Design review of the part built by this model. Coordinates are the model's own, in mm. A direction names the side the tool comes from. Round coordinates to 2 decimals unless told otherwise and drop trailing zeros. Write each loop counter-clockwise with the first axis right and the second up, starting at its lowest first coordinate (ties: lowest second). Pieces come first, ordered by that corner, then holes. Notation, with made-up numbers: (40, -3.75) -> (45, -3.75) arc R24 cw to (45, 11.25) -> close; hole circle Ø4 at (44, 62). An arc over 180 degrees is marked (long way). One line per question, with ' | ' between items. Start each with the question number.
1) Insertion check: pin 1 Ø1.2 at (y, z) = (5, -8.5) entering from +X; pin 2 Ø3.5 at (x, y) = (-3, 4.5) entering from +Z; pin 3 Ø3.5 at (y, z) = (8, -3) entering from -X. Each pin has a flat end and moves straight along its axis. Give the tip position at first contact, or say it passes through.
2) Consider section C-C (x = 25.4). Give the boundary of the cut face in (y, z).
3) Consider section A-A (y = 6.35). Give the boundary of the cut face in (x, z).
4) Mouldability with a two-part tool opening along Y and no side actions: class faces 5 (the flat face through (-20, 6, -11.049)), 6 (the flat face through (0, 0, -7)), 7 (the cylindrical face through (22.025, 6.499, -12.614)) as +Y half, -Y half, draft (parallel to the pull), parting line (faces both ways), or undercut.
5) Consider section D-D (z = -4.75). Give the boundary of the cut face in (x, y), then the cut area to 3 significant figures.
6) For probe 1 along Y at (x, z) = (25.4, -13.1); probe 2 along X at (y, z) = (7.75, 0); probe 3 along Z at (x, y) = (-1.5, 11.5), list the stretches that pass through material, from the lowest coordinate up.
7) Consider section B-B (x = 0). Give the boundary of the cut face in (y, z), then the cut area to 3 significant figures.
8) For faces 1 (the flat face through (9.271, 6, -6)), 2 (the cylindrical face through (0.2, 6.26, 9.27)), 3 (the flat face through (-9.271, 6, -5)), 4 (the flat face through (-6.096, 6, -9)), list the 3-axis set-ups (+Z, -Z, +X, -X, +Y, -Y) from which the entire face can be reached by the end or side of a thin tool; tool diameter is ignored.
```python
from build123d import *

# Parameters (mm, degrees)
SKETCH1_R           = 6.096
BOSS_EXTRUDE1_DEPTH = 12.7
SKETCH2_R           = 3.3782
CUT_EXTRUDE1_DEPTH  = 4.175


with BuildPart() as part:
    # Sketch1 → Boss-Extrude1 (new body)
    with BuildSketch(Plane(origin=(0, 0, 0), x_dir=(1, 0, 0), z_dir=(0, 1, 0))):
        with BuildLine():
            Line((-9.271, 0), (-9.271, 11.049))
            Line((-9.271, 11.049), (-31.496, 11.049))
            Line((-31.496, 11.049), (-31.496, 14.224))
            Line((-31.496, 14.224), (-6.096, 14.224))
            Line((-6.096, 14.224), (6.096, 14.224))
            Line((6.096, 14.224), (31.496, 14.224))
            Line((31.496, 14.224), (31.496, 11.049))
            Line((31.496, 11.049), (9.271, 11.049))
            Line((9.271, 11.049), (9.271, 0))
            ThreePointArc((9.271, 0), (0, -9.271), (-9.271, 0))
        make_face()
        Circle(SKETCH1_R, mode=Mode.SUBTRACT)
        with BuildLine():
            Line((-6.096, 7.112), (-6.096, 11.049))
            Line((-6.096, 11.049), (6.096, 11.049))
            Line((6.096, 11.049), (6.096, 7.112))
            ThreePointArc((6.096, 7.112), (0, 9.367057169), (-6.096, 7.112))
        make_face(mode=Mode.SUBTRACT)
    extrude(amount=BOSS_EXTRUDE1_DEPTH)

    # Sketch2 → Cut-Extrude1 (cut, through all)
    with BuildSketch(Plane.XY.offset(-11.049)):
        with Locations((-25.4, 6.35)):
            Circle(SKETCH2_R)
        with Locations((25.4, 6.35)):
            Circle(SKETCH2_R)
    extrude(amount=-CUT_EXTRUDE1_DEPTH, mode=Mode.SUBTRACT)


solid = part.part
```
From the geometry:
1) pin 1: stops at x = 9.27 | pin 2: stops at z = 9.19 | pin 3: stops at x = -9.27
2) outline: (0, -14.22) -> (2.97, -14.22) -> (2.97, -11.05) -> (0, -11.05) -> close; (9.73, -14.22) -> (12.7, -14.22) -> (12.7, -11.05) -> (9.73, -11.05) -> close
3) outline: (-31.5, -14.22) -> (-28.78, -14.22) -> (-28.78, -11.05) -> (-31.5, -11.05) -> close; (-22.02, -14.22) -> (22.02, -14.22) -> (22.02, -11.05) -> (9.27, -11.05) -> (9.27, 0) arc R9.27 ccw to (-9.27, 0) -> (-9.27, -11.05) -> (-22.02, -11.05) -> close; (28.78, -14.22) -> (31.5, -14.22) -> (31.5, -11.05) -> (28.78, -11.05) -> close; hole (-6.1, -11.05) -> (6.1, -11.05) -> (6.1, -7.11) arc R9.37 cw to (-6.1, -7.11) -> close; hole circle Ø12.19 at (0, 0)
4) face 5: draft | face 6: -Y half | face 7: undercut
5) outline: (-9.27, 0) -> (-3.82, 0) -> (-3.82, 12.7) -> (-9.27, 12.7) -> close; (3.82, 0) -> (9.27, 0) -> (9.27, 12.7) -> (3.82, 12.7) -> close | area: 138 mm2
6) probe 1: y = 0 to 2.97, 9.73 to 12.7 | probe 2: x = -9.27 to -6.1, 6.1 to 9.27 | probe 3: z = -14.22 to -11.05, -9.25 to -5.91, 5.91 to 9.15
7) outline: (0, -14.22) -> (12.7, -14.22) -> (12.7, -11.05) -> (0, -11.05) -> close; (0, -9.37) -> (12.7, -9.37) -> (12.7, -6.1) -> (0, -6.1) -> close; (0, 6.1) -> (12.7, 6.1) -> (12.7, 9.27) -> (0, 9.27) -> close | area: 122 mm2
8) face 1: +Z, +X, +Y, -Y | face 2: +Z, +Y, -Y | face 3: +Z, -X, +Y, -Y | face 4: +Y, -Y
